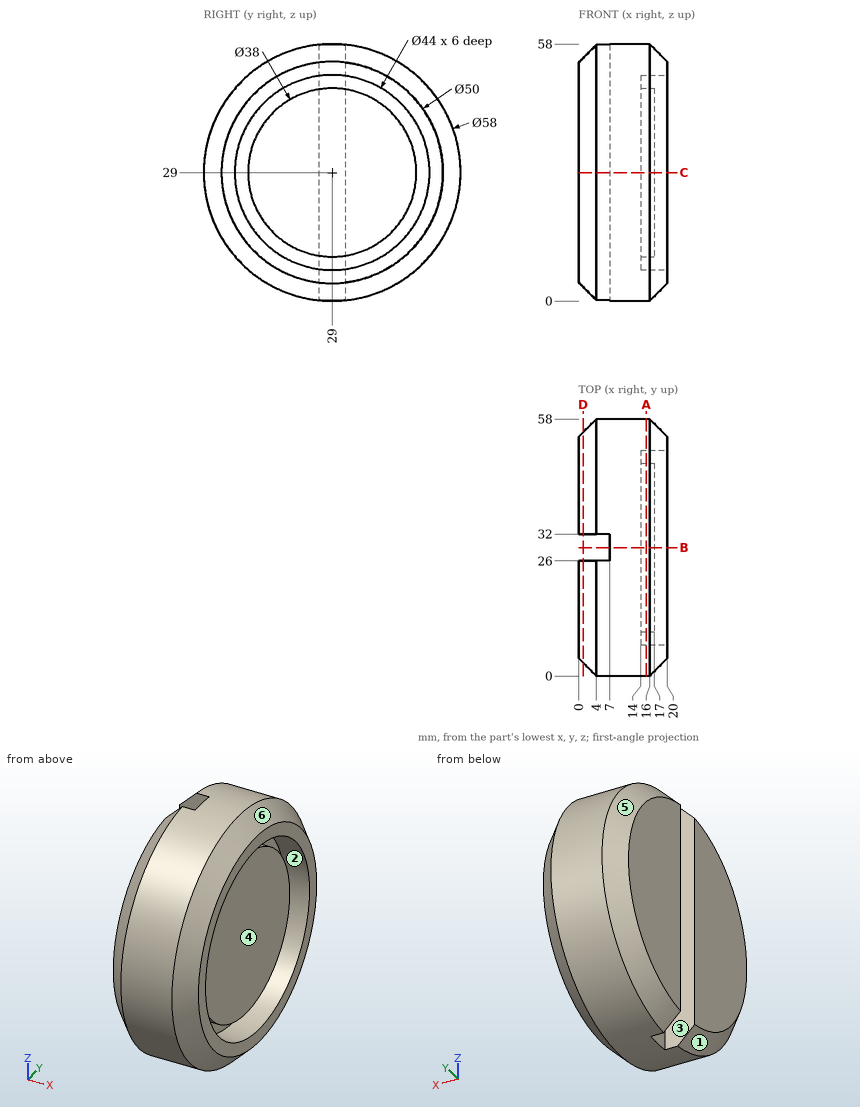
Verification items for this drawing (mm, ordinates from the low corner). A direction names the side the tool comes from. Coordinates: 2 decimals unless noted, no trailing zeros. Loops run counter-clockwise (first coordinate to the right, second up) from the corner with the lowest first, then second, coordinate; pieces in that order, holes last. Notation, with made-up numbers: (27, 61) -> (34, 61) arc R23 ccw to (34, 87) -> close; hole circle Ø7 at (-3, 64). An arc over 180 degrees is marked (long way). Answer in a Markdown table with one row per item. Add a question column.
1. Depth check by flat-ended pin: P1, Ø1, axis at x = 3, z = 21, coming from the +Y side; P2, Ø7.5, axis at x = 2.5, z = 24, coming from the +Y side; P3, Ø5, axis at x = 14, y = 29, coming from the -Z side; P4, Ø10, axis at y = 42.5, z = 6, coming from the -X side. Enter the tip coordinate at first touch or a pass-through.
2. Access from +Z, -Z, +X, -X, +Y, -Y to the whole of each face (thin tool, end or side, straight path). Record for the marked faces 1 and 2.
3. Section check D-D, the plane x = 1. Enter the section's corners in (y, z), then the cut area to 3 significant figures.
4. Draft check along Y on the marked faces 3, 4, 5 and 6. Enter one of: +Y half, -Y half, draft (parallel to the pull), parting line (faces both ways), or undercut.
5. Section check C-C, the plane z = 29. Enter the section's corners in (x, y).
6. Section check B-B, the plane y = 29. Enter the section's corners in (x, z).
7. Material ranges on probe 1 along Z at (x, y) = (15.9, 29); probe 2 along X at (y, z) = (45, 31); probe 3 along Y at (x, z) = (6.75, 50), recorded low to high. Write a range as [from, to].
8. Section check A-A, the plane x = 15.25. Enter the section's corners in (y, z).
Derived:
| question | item | result |
|---|---|---|
| 1 | P1 | stops at y = 56.37 |
| 1 | P2 | stops at y = 57.96 |
| 1 | P3 | stops at z = 0 |
| 1 | P4 | stops at x = 0 |
| 2 | face 1 | -X, -Y |
| 2 | face 2 | +X |
| 3 | outline | (26, 3.17) -> (26, 54.83) arc R26 ccw to start; (32, 3.17) arc R26 ccw to (32, 54.83) -> close |
| 3 | area | 1,810 mm² |
| 4 | face 3 | undercut |
| 4 | face 4 | undercut |
| 4 | face 5 | +Y half |
| 4 | face 6 | parting line |
| 5 | outline | (0, 4) -> (4, 0) -> (16, 0) -> (20, 4) -> (20, 7) -> (14, 7) -> (14, 10) -> (17, 10) -> (17, 48) -> (14, 48) -> (14, 51) -> (20, 51) -> (20, 54) -> (16, 58) -> (4, 58) -> (0, 54) -> (0, 32) -> (7, 32) -> (7, 26) -> (0, 26) -> close |
| 6 | outline | (7, 0) -> (16, 0) -> (20, 4) -> (20, 7) -> (14, 7) -> (14, 10) -> (17, 10) -> (17, 48) -> (14, 48) -> (14, 51) -> (20, 51) -> (20, 54) -> (16, 58) -> (7, 58) -> close |
| 7 | probe 1 | z = [0, 7], [10, 48], [51, 58] |
| 7 | probe 2 | x = [0, 17] |
| 7 | probe 3 | y = [9, 26], [32, 49] |
| 8 | outline | circle Ø58 at (29, 29); circle Ø38 at (29, 29); hole circle Ø44 at (29, 29) |
